```python
from build123d import *

# Parameters (mm, degrees)
F0_W     = 235
F0_H     = 170
F1_DEPTH = 5
F2_W     = 235
F2_H     = 170
F2_W_2   = 110
F2_H_2   = 50
F3_DEPTH = 10


with BuildPart() as f1:
    # F0 (on Top) → F1 (new body)
    with BuildSketch(Plane.XY):
        Rectangle(F0_W, F0_H)
    extrude(amount=F1_DEPTH)

    # F2 (on face) → F3 (join)
    with BuildSketch(Plane.XY.offset(5)):
        Rectangle(F2_W, F2_H)
        with Locations((-57.5, -55)):
            Rectangle(F2_W_2, F2_H_2, mode=Mode.SUBTRACT)
        with Locations((57.5, -55)):
            Rectangle(F2_W_2, F2_H_2, mode=Mode.SUBTRACT)
        with Locations((-57.5, 0)):
            Rectangle(F2_W_2, F2_H_2, mode=Mode.SUBTRACT)
        with Locations((-57.5, 55)):
            Rectangle(F2_W_2, F2_H_2, mode=Mode.SUBTRACT)
        with Locations((57.5, 0)):
            Rectangle(F2_W_2, F2_H_2, mode=Mode.SUBTRACT)
        with Locations((57.5, 55)):
            Rectangle(F2_W_2, F2_H_2, mode=Mode.SUBTRACT)
    extrude(amount=F3_DEPTH)


solid = f1.part
```
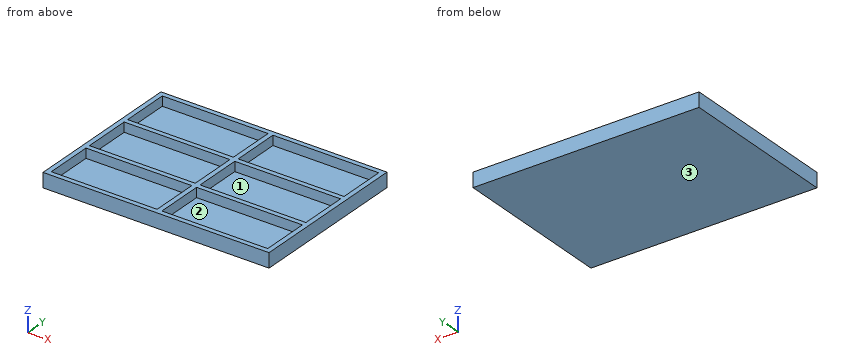
Check sheet for the modelled part. Datum: model origin and axes. Units: mm. Face numbers are marked on the shaded views. Coordinates: 2 decimals unless noted, no trailing zeros. Loops run counter-clockwise (first coordinate to the right, second up) from the corner with the lowest first, then second, coordinate; pieces in that order, holes last.
1) Release check for a two-part mould opening along Y. For the marked faces 1, 2 and 3 record: released by +Y, released by -Y, zero draft, split by the parting line, or undercut.
2) Sectioned sample at C-C (x = -75). Record the boundary of the cut face in (y, z).
3) Gauge pin test, flat ends, axial feed: pin 1 (10 mm diameter, centred on x = 84.5, y = -16.5, fed in from -Z); pin 2 (25 mm diameter, centred on x = -77, y = -56.5, fed in from +Z). Record the tip position at first contact, or that the pin passes through.
4) Sectioned sample at A-A (y = 2.5). Record the boundary of the cut face in (x, z), and give its area (4 significant figures).
5) Sectioned sample at B-B (z = 8.75). Record the boundary of the cut face in (x, y).
6) Material ranges on probe 1 along Y at (x, z) = (-96.5, 9); probe 2 along X at (y, z) = (4, 10.5); probe 3 along Z at (x, y) = (-88, -23.5), recorded low to high.
Check sheet entries:
1. face 1: undercut
1. face 2: undercut
1. face 3: zero draft
2. outline: (-85, 0) - (85, 0) - (85, 15) - (80, 15) - (80, 5) - (30, 5) - (30, 15) - (25, 15) - (25, 5) - (-25, 5) - (-25, 15) - (-30, 15) - (-30, 5) - (-80, 5) - (-80, 15) - (-85, 15) - close
3. pin 1: stops at z = 0
3. pin 2: stops at z = 5
4. outline: (-117.5, 0) - (117.5, 0) - (117.5, 15) - (112.5, 15) - (112.5, 5) - (2.5, 5) - (2.5, 15) - (-2.5, 15) - (-2.5, 5) - (-112.5, 5) - (-112.5, 15) - (-117.5, 15) - close
4. area: 1,325 mm2
5. outline: (-117.5, -85) - (117.5, -85) - (117.5, 85) - (-117.5, 85) - close; hole (-112.5, -80) - (-2.5, -80) - (-2.5, -30) - (-112.5, -30) - close; hole (-112.5, -25) - (-2.5, -25) - (-2.5, 25) - (-112.5, 25) - close; hole (-112.5, 30) - (-2.5, 30) - (-2.5, 80) - (-112.5, 80) - close; hole (2.5, -80) - (112.5, -80) - (112.5, -30) - (2.5, -30) - close; hole (2.5, -25) - (112.5, -25) - (112.5, 25) - (2.5, 25) - close; hole (2.5, 30) - (112.5, 30) - (112.5, 80) - (2.5, 80) - close
6. probe 1: y = -85 to -80, -30 to -25, 25 to 30, 80 to 85
6. probe 2: x = -117.5 to -112.5, -2.5 to 2.5, 112.5 to 117.5
6. probe 3: z = 0 to 5
